Here's the drawing with two shaded views (mm, measured from the low corner). I have some questions. Round coordinates to 2 decimals unless told otherwise and drop trailing zeros. Write each loop counter-clockwise with the first axis right and the second up, starting at its lowest first coordinate (ties: lowest second). Pieces come first, ordered by that corner, then holes. Notation, with made-up numbers: M 88,59 L 96,59 A29 cw 96,80 Z; hole C -36.5,54.25 d11. An arc over 180 degrees is marked long. Write item = value, one per line. Start each with the question number.
(1) If we mould it in two halves opening along X, with no side actions, what happens to the marked faces 1 and 2? For each: released by +X, released by -X, zero draft, split by the parting line, or undercut.
(2) Will these pins go through, and if not, where does the flat tip stop? pin 1 Ø0.9 at (x, z) = (1, 5.5) entering from +Y; pin 2 Ø3 at (y, z) = (1.5, 26) entering from +X; pin 3 Ø0.5 at (x, y) = (1.5, 0.5) entering from +Z; pin 4 Ø1.9 at (x, z) = (83.5, 65) entering from -Y.
(3) I want a section at A-A (y = 1.85). List the corners of the cut face in (x, z) for me.
(4) I want a section at C-C (z = 65). List the corners of the cut face in (x, y) for me, and give its area (3 significant figures).
(5) I want a section at B-B (x = 1.5). List the corners of the cut face in (y, z) for me, and give its area (3 significant figures).
(6) I want a section at D-D (z = 24). List the corners of the cut face in (x, y) for me.
(7) I need wall thicknesses on line 1 along X through (y, z) = (0.7, 5); line 2 along Z through (x, y) = (83.5, 0.7); line 3 along X through (y, z) = (1.2, 56.5). Which ranges of each line are inside material? Lowest first, please.
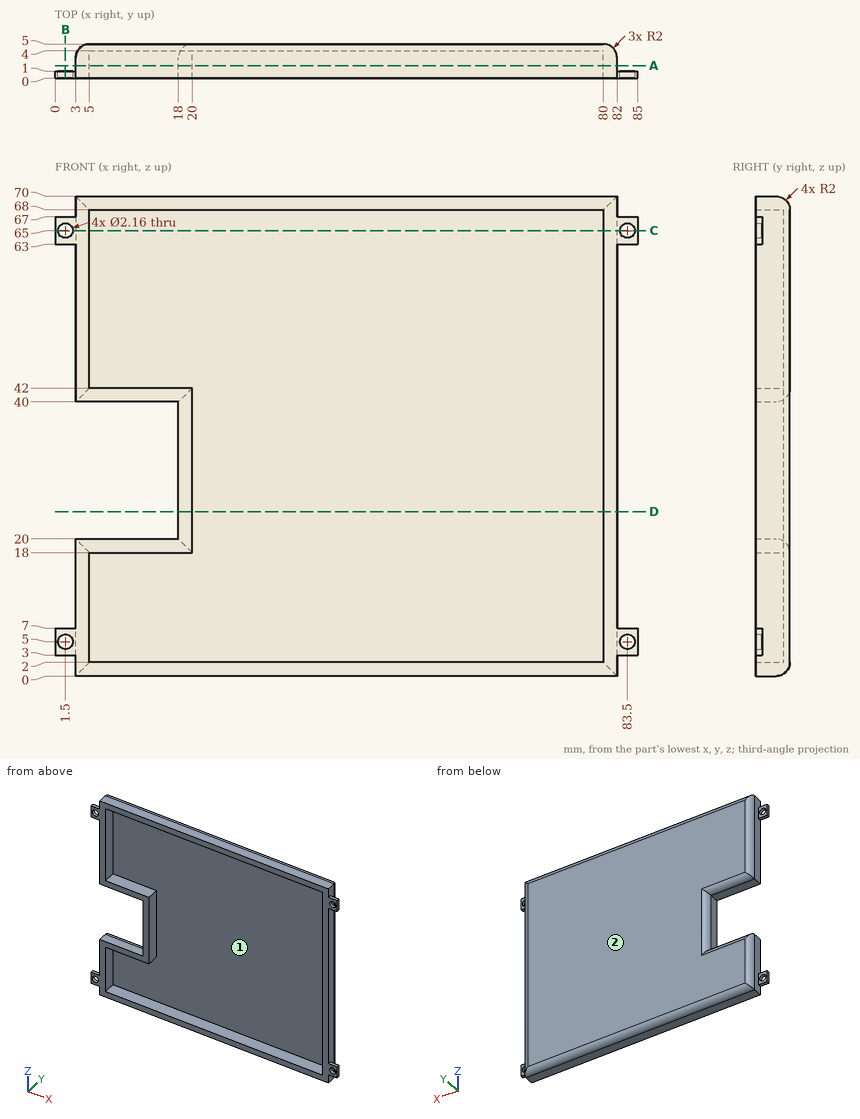
Returned:
q1.face_1 = undercut
q1.face_2 = zero draft
q2.pin_1 = 1
q2.pin_2 = 82
q2.pin_3 = 67
q2.pin_4 = through
q3.outline = M 3,0 L 82,0 L 82,70 L 3,70 L 3,40 L 18,40 L 18,20 L 3,20 Z; hole M 5,2 L 80,2 L 80,68 L 5,68 L 5,42 L 20,42 L 20,18 L 5,18 Z
q4.outline = M 0,0 L 0.42,0 L 0.42,1 L 0,1 Z; M 2.58,0 L 5,0 L 5,4 L 80,4 L 80,0 L 82.42,0 L 82.42,1 L 82,1 L 82,3 A2 ccw 80,5 L 5,5 A2 ccw 3,3 L 3,1 L 2.58,1 Z; M 84.58,0 L 85,0 L 85,1 L 84.58,1 Z
q4.area = 95.0 mm²
q5.outline = M 0,3 L 1,3 L 1,3.92 L 0,3.92 Z; M 0,6.08 L 1,6.08 L 1,7 L 0,7 Z; M 0,63 L 1,63 L 1,63.92 L 0,63.92 Z; M 0,66.08 L 1,66.08 L 1,67 L 0,67 Z
q5.area = 3.68 mm²
q6.outline = M 18,0 L 20,0 L 20,4 L 80,4 L 80,0 L 82,0 L 82,3 A2 ccw 80,5 L 20,5 A2 ccw 18,3 Z
q7.line_1 = 0 to 0.42, 2.58 to 5, 80 to 82.42, 84.58 to 85
q7.line_2 = 3 to 3.92, 6.08 to 7, 63 to 63.92, 66.08 to 67
q7.line_3 = 3 to 5, 80 to 82
